```python
from build123d import *

# Parameters (mm, degrees)
BOSS_EXTRUDE1_DEPTH = 15
FILLET1_R           = 4
SHELL1_T            = 2


with BuildPart() as part:
    # Sketch1 → Boss-Extrude1 (new, symmetric)
    with BuildSketch(Plane(origin=(0, 0, 0), x_dir=(1, 0, 0), z_dir=(0, 1, 0))):
        with BuildLine():
            Line((-74, 59.5), (74, 59.5))
            ThreePointArc((74, 59.5), (79.656854249, 57.156854249), (82, 51.5))
            Line((82, 51.5), (82, -51.5))
            ThreePointArc((82, -51.5), (79.656854249, -57.156854249), (74, -59.5))
            Line((74, -59.5), (-74, -59.5))
            ThreePointArc((-74, -59.5), (-79.656854249, -57.156854249), (-82, -51.5))
            Line((-82, -51.5), (-82, 51.5))
            ThreePointArc((-82, 51.5), (-79.656854249, 57.156854249), (-74, 59.5))
        make_face()
    extrude(amount=BOSS_EXTRUDE1_DEPTH, both=True)

    # Fillet1
    fillet1_edges = [part.edges().sort_by_distance(p)[0] for p in [
        (-79.656854249, -15, -57.156854249),
        (-82, -15, 0),
        (-79.656854249, -15, 57.156854249),
        (0, -15, 59.5),
        (79.656854249, -15, 57.156854249),
        (82, -15, 0),
        (79.656854249, -15, -57.156854249),
        (0, -15, -59.5),
    ]]
    fillet(fillet1_edges, radius=FILLET1_R)

    # Shell1
    shell1_openings = [part.faces().sort_by_distance(p)[0] for p in [
        (0, 15, 0),
    ]]
    offset(amount=SHELL1_T, openings=shell1_openings, kind=Kind.INTERSECTION)


solid = part.part
```
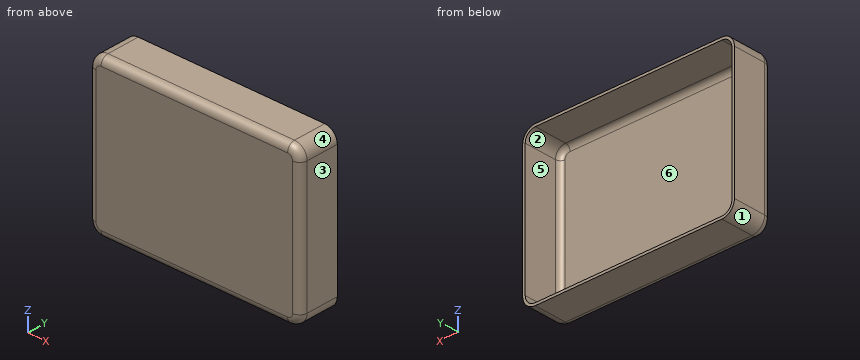
Input: part model. Units: mm. Frame: model coordinates. Face numbers are marked on the shaded views. A direction names the side the tool comes from. Coordinates: 2 decimals unless noted, no trailing zeros. Write each loop counter-clockwise with the first axis right and the second up, starting at its lowest first coordinate (ties: lowest second). Pieces come first, ordered by that corner, then holes. Notation, with made-up numbers: (84, 74.5) -> (120, 74.5) arc R33 cw to (120, 106.5) -> close; hole circle Ø5 at (27, -17). An arc over 180 degrees is marked (long way). Write each question's results on one line, items separated by ' | '.
Item 1: Set-up query: the marked faces 1 and 2. Return all of +Z, -Z, +X, -X, +Y, -Y with unobstructed straight access to the full face (end or side cutting, diameter ignored); none if empty.
Conclusion:
face 1: -Z, -X, +Y, -Y | face 2: +Y
Item 2: Section query A-A on y = -0.5. Return loops of the section in (x, z), plus the area to 3 significant figures.
Conclusion:
outline: (-84, -51.5) arc R10 ccw to (-74, -61.5) -> (74, -61.5) arc R10 ccw to (84, -51.5) -> (84, 51.5) arc R10 ccw to (74, 61.5) -> (-74, 61.5) arc R10 ccw to (-84, 51.5) -> close; hole (-82, -51.5) arc R8 ccw to (-74, -59.5) -> (74, -59.5) arc R8 ccw to (82, -51.5) -> (82, 51.5) arc R8 ccw to (74, 59.5) -> (-74, 59.5) arc R8 ccw to (-82, 51.5) -> close | area: 1,120 mm^2
Item 3: Section query B-B on z = -34.5. Return loops of the section in (x, y), plus the area to 3 significant figures.
Conclusion:
outline: (-84, -11) arc R6 ccw to (-78, -17) -> (78, -17) arc R6 ccw to (84, -11) -> (84, 15) -> (82, 15) -> (82, -11) arc R4 cw to (78, -15) -> (-78, -15) arc R4 cw to (-82, -11) -> (-82, 15) -> (-84, 15) -> close | area: 447 mm^2
Item 4: Mould query, pull axis Z, two halves, no side actions, for the marked faces 3, 4, 5 and 6. Classes: +Z half, -Z half, draft (parallel to the pull), parting line (faces both ways), or undercut.
Conclusion:
face 3: draft | face 4: +Z half | face 5: undercut | face 6: undercut
Item 5: Pin query (flat end, axial travel): pin 1 Ø1.5 at (x, z) = (59, -47) entering from +Y. Return the tip coordinate at first contact, or that it passes through.
Conclusion:
pin 1: stops at y = -15
Item 6: Material intervals for probe 1 along X at (y, z) = (12.5, 34); probe 2 along Z at (x, y) = (12, 10); probe 3 along Y at (x, z) = (0, 38), sorted ascending.
Conclusion:
probe 1: x = -84 to -82, 82 to 84 | probe 2: z = -61.5 to -59.5, 59.5 to 61.5 | probe 3: y = -17 to -15
Item 7: Section query C-C on x = 60.5. Return loops of the section in (y, z).
Conclusion:
outline: (-17, -55.5) arc R6 ccw to (-11, -61.5) -> (15, -61.5) -> (15, -59.5) -> (-11, -59.5) arc R4 cw to (-15, -55.5) -> (-15, 55.5) arc R4 cw to (-11, 59.5) -> (15, 59.5) -> (15, 61.5) -> (-11, 61.5) arc R6 ccw to (-17, 55.5) -> close
